Source: CAD feature listing. Evaluate the final solid. Frame: model axes, mm. A direction names the side the tool comes from. Round coordinates to 2 decimals unless told otherwise and drop trailing zeros. Loops run counter-clockwise (first coordinate to the right, second up) from the corner with the lowest first, then second, coordinate; pieces in that order, holes last.
(1) Section B-B, the plane y = 38.5. Return the cut outline in (x, z), plus the area to 3 significant figures.
(2) Material intervals for probe 1 along Y at (x, z) = (0, 2.75); probe 2 along Y at (x, z) = (6, 5.75); probe 3 along X at (y, z) = (-21, 4.5), sorted ascending.
(3) Section D-D, the plane z = 2.5. Return the cut outline in (x, y), plus the area to 3 significant figures.
(4) Set-up query: faces 4 (the flat face through (-18.7, -27.767, 3.451)), 5 (the flat face through (39.077, -22.307, 3.451)). Return all of +Z, -Z, +X, -X, +Y, -Y with unobstructed straight access to the full face (end or side cutting, diameter ignored); none if empty.
(5) Section A-A, the plane x = 0. Return the cut outline in (y, z).
(6) First-contact query: pin 1 Ø4 at (y, z) = (-6.5, 1.5) entering from +X; pin 2 Ø4 at (y, z) = (-1.5, 3) entering from +X. Flat tips, straight axial feed; report the tip coordinate or a pass-through.
(7) Mould query, pull axis X, two halves, no side actions, for faces 1 (the cylindrical face through (15.03, 9.06, 3.45)), 2 (the cylindrical face through (-11.19, 0.49, 3.45)), 3 (the flat face through (-33.78, -2.53, 3.45)). Classes: pulls with the +X half, pulls with the -X half, needs draft (parallel to the pull), parting line crosses it, or undercut.
(8) Section C-C, the plane x = -33.5. Return the cut outline in (y, z), plus the area to 3 significant figures.
```python
from build123d import *

# Parameters (mm, degrees)
F0_R     = 11.2
F1_DEPTH = 7


with BuildPart() as f1:
    # F0 (on Top) → F1 (new body)
    with BuildSketch(Plane.XY):
        with BuildLine():
            Line((14.265774, 45.414708), (-15.116394, 44.564087))
            Line((-15.116394, 44.564087), (-14.265774, 15.181919))
            ThreePointArc((-14.265774, 15.181919), (-15.420315, 8.400052), (-21.442784, 5.074912))
            Line((-21.442784, 5.074912), (-46.463177, -10.352831))
            Line((-46.463177, -10.352831), (-31.035434, -35.373225))
            Line((-31.035434, -35.373225), (-6.01504, -19.945482))
            ThreePointArc((-6.01504, -19.945482), (0.435499, -17.554411), (6.326389, -21.107451))
            Line((6.326389, -21.107451), (32.197404, -35.061876))
            Line((32.197404, -35.061876), (46.151829, -9.190862))
            Line((46.151829, -9.190862), (20.280814, 4.763563))
            ThreePointArc((20.280814, 4.763563), (14.984816, 9.154359), (15.116394, 16.032539))
            Line((15.116394, 16.032539), (14.265774, 45.414708))
        make_face()
        with Locations((-26.239109, -15.149157)):
            Circle(F0_R, mode=Mode.SUBTRACT)
        Circle(F0_R, mode=Mode.SUBTRACT)
        with Locations((26.239109, -15.149157)):
            Circle(F0_R, mode=Mode.SUBTRACT)
        with Locations((0, 30.298313)):
            Circle(F0_R, mode=Mode.SUBTRACT)
    extrude(amount=F1_DEPTH)


solid = f1.part
```
Output values:
1. outline: (-14.94, 0) - (-7.63, 0) - (-7.63, 7) - (-14.94, 7) - close; (7.63, 0) - (14.47, 0) - (14.47, 7) - (7.63, 7) - close
1. area: 99.1 mm2
2. probe 1: y = -17.53 to -11.2, 11.2 to 19.1, 41.5 to 45
2. probe 2: y = -20.65 to -9.46, 9.46 to 20.84, 39.76 to 45.18
2. probe 3: x = -39.9 to -35.79, -16.69 to -7.73, 6.25 to 16.69, 35.79 to 39.78
3. outline: (-46.46, -10.35) - (-31.04, -35.37) - (-6.02, -19.95) arc R7.93 cw to (6.33, -21.11) - (32.2, -35.06) - (46.15, -9.19) - (20.28, 4.76) arc R7.93 cw to (15.12, 16.03) - (14.27, 45.41) - (-15.12, 44.56) - (-14.27, 15.18) arc R7.93 cw to (-21.44, 5.07) - close; hole circle Ø22.4 at (-26.24, -15.15); hole circle Ø22.4 at (0, 0); hole circle Ø22.4 at (0, 30.3); hole circle Ø22.4 at (26.24, -15.15)
3. area: 2,010 mm2
4. face 4: +Z, -Z, -Y
4. face 5: +Z, -Z, +X, -Y
5. outline: (-17.53, 0) - (-11.2, 0) - (-11.2, 7) - (-17.53, 7) - close; (11.2, 0) - (19.1, 0) - (19.1, 7) - (11.2, 7) - close; (41.5, 0) - (45, 0) - (45, 7) - (41.5, 7) - close
6. pin 1: stops at x = 44.87
6. pin 2: stops at x = 35.6
7. face 1: pulls with the +X half
7. face 2: undercut
7. face 3: pulls with the -X half
8. outline: (-31.38, 0) - (-23.68, 0) - (-23.68, 7) - (-31.38, 7) - close; (-6.62, 0) - (-2.36, 0) - (-2.36, 7) - (-6.62, 7) - close
8. area: 83.7 mm2
